Could you check a few things on this drawing? It's one solid part, dimensions in mm from its lowest x, y, z. A direction names the side the tool comes from. Give positions to 0.01 mm unless a question says otherwise; leave off trailing zeros. Write each loop counter-clockwise with the first axis right and the second up, starting at its lowest first coordinate (ties: lowest second). Pieces come first, ordered by that corner, then holes. Notation, with made-up numbers: (4, 15.5) - (51, 15.5) arc R23 ccw to (51, 25.5) - close; hole circle Ø9 at (71, -9). An arc over 180 degrees is marked (long way). One line per item, written item: value. Start each with the question number.
1) Imagine slicing it at C-C on x = 5. Write out the boundary of the cut face in (y, z).
2) Imagine slicing it at B-B on x = 28. Write out the boundary of the cut face in (y, z).
3) Imagine slicing it at A-A on z = 6.5. Write out the boundary of the cut face in (x, y).
4) We'd pull the mould along X, two halves only. Please class the marked faces 1, 2 and 3: +X half, -X half, draft (parallel to the pull), parting line (faces both ways), or undercut.
5) On a 3-axis mill with a long thin cutter (end or side, diameter ignored), from which of +Z, -Z, +X, -X, +Y, -Y can I reach the whole of each face in a straight line? I mean the marked faces 4, 5 and 6. Say none if no direction works.
6) I'm going to push flat-ended pins straight in: P1, Ø0.6, axis at x = 20.5, z = 25, coming from the +Y side; P2, Ø1.6, axis at x = 37, z = 24.5, coming from the +Y side; P3, Ø6, axis at x = 28.5, z = 16, coming from the +Y side. Where does each tip first touch, or does it pass through?
7) Imagine slicing it at D-D on y = 26. Write out the boundary of the cut face in (x, z).
8) Please list where these lines run through material, in increasing order: L1, parallel to Z at x = 36.5, y = 11.5; L2, parallel to X at y = 21.5, z = 8.25; L3, parallel to Y at x = 38.5, z = 23.25. Write a range as [from, to].
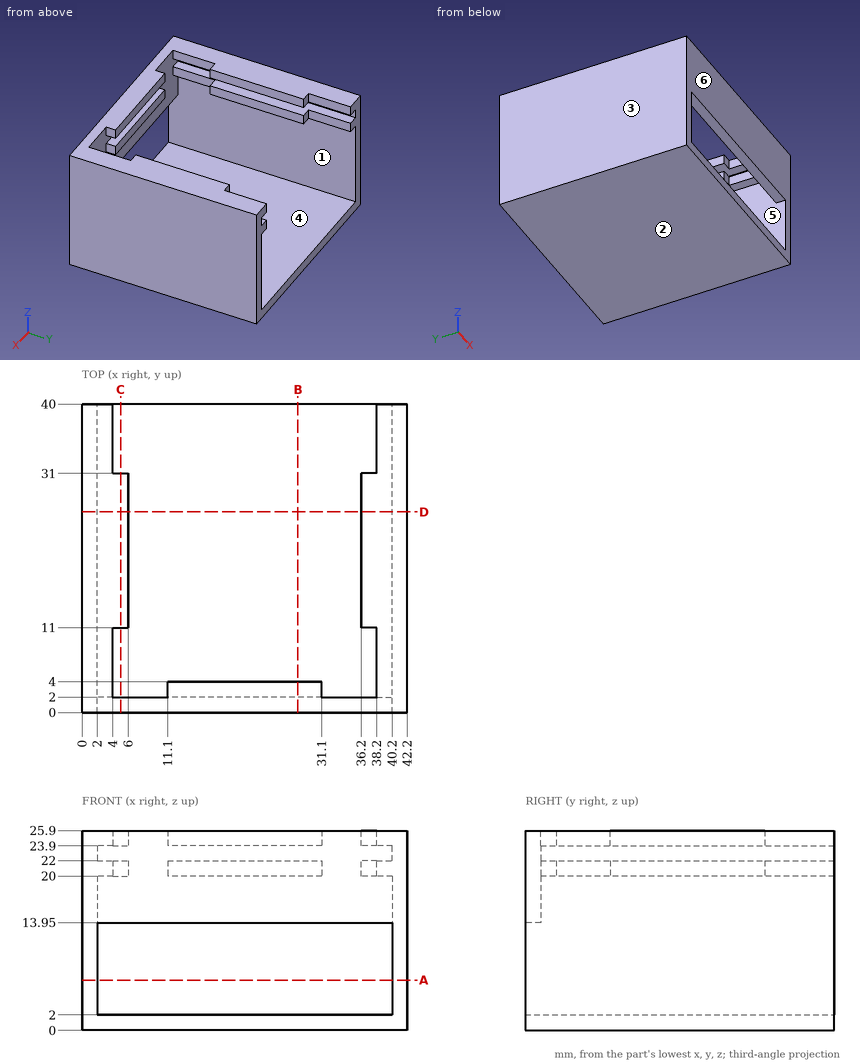
Numbers:
1. outline: (0, 0) - (40, 0) - (40, 2) - (0, 2) - close; (0, 13.95) - (2, 13.95) - (2, 25.9) - (0, 25.9) - close; (11, 20) - (31, 20) - (31, 22) - (11, 22) - close; (11, 23.9) - (31, 23.9) - (31, 25.9) - (11, 25.9) - close
2. outline: (0, 0) - (40, 0) - (40, 2) - (0, 2) - close; (0, 13.95) - (2, 13.95) - (2, 20) - (4, 20) - (4, 22) - (2, 22) - (2, 23.9) - (4, 23.9) - (4, 25.9) - (0, 25.9) - close
3. outline: (0, 0) - (2, 0) - (2, 40) - (0, 40) - close; (40.2, 0) - (42.2, 0) - (42.2, 40) - (40.2, 40) - close
4. face 1: undercut
4. face 2: draft
4. face 3: -X half
5. face 4: +Y, -Y
5. face 5: +Y
5. face 6: +Z, -Z, +X, -X, -Y
6. P1: y = 4
6. P2: y = 31
6. P3: y = 2
7. outline: (0, 0) - (42.2, 0) - (42.2, 25.9) - (36.2, 25.9) - (36.2, 23.9) - (40.2, 23.9) - (40.2, 22) - (36.2, 22) - (36.2, 20) - (40.2, 20) - (40.2, 2) - (2, 2) - (2, 20) - (6, 20) - (6, 22) - (2, 22) - (2, 23.9) - (6, 23.9) - (6, 25.9) - (0, 25.9) - close
8. L1: [0, 2], [20, 22], [23.9, 25.9]
8. L2: [0, 2], [40.2, 42.2]
8. L3: [0, 2]
